Check sheet for the modelled part. Datum: model origin and axes. Units: mm. A direction names the side the tool comes from. Round coordinates to 2 decimals unless told otherwise and drop trailing zeros. Write each loop counter-clockwise with the first axis right and the second up, starting at its lowest first coordinate (ties: lowest second). Pieces come first, ordered by that corner, then holes.
Item 1: Cross-section at C-C on y = -2.5. Enter the section's corners in (x, z).
Item 2: Tool access check on faces 4 (the cylindrical face through (-0.867, -3.905, -0.246)), 5 (the flat face through (1.3, -1.3, 1)), 6 (the flat face through (2, 0, -0.5)). Record the directions out of +Z, -Z, +X, -X, +Y, -Y that give a thin tool (end or side, any length) a straight path to the whole face; none if there is none.
Item 3: Go/stop test with flat-tipped pins: pin 1 Ø1.5 at (x, z) = (3.5, 8.5) entering from -Y; pin 2 Ø3 at (x, y) = (1, -0.5) entering from +Z; pin 3 Ø2 at (x, z) = (4, 2.5) entering from -Y. Record where each tip stops, or that it passes through.
Item 4: Cross-section at A-A on y = -0.5. Enter the section's corners in (x, z), plus the area to 3 significant figures.
Item 5: Release check for a two-part mould opening along Y. For faces 1 (the cylindrical face through (-1.653, 2.593, 5.338)), 2 (the cylindrical face through (0, 5, 5)), 3 (the flat face through (0.1, 3.3, 9.8)) record: +Y half, -Y half, draft (parallel to the pull), parting line (faces both ways), or undercut.
Item 6: Material ranges on line 1 (Y direction, x = 0, z = 0.15); line 2 (Y direction, x = 0, z = -0.05), recorded low to high.
Autodesk Fusion 360 part; units mm, degrees
sketch "Sketch1" plane through (0, 0, 0) normal (0, 0, 1) x (1, 0, 0)
  circle A0 centre (0, 0) radius 5
  circle A1 centre (0, 0) radius 1.65
  dimension "d1" = 10
  dimension "d2" = 3.3
extrude "Extrude1" add sketch "Sketch1" along normal blind 1
sketch "Sketch2" plane through (0, 0, 1) normal (0, 0, 1) x (-1, 0, 0)
  circle A0 centre (0, 0) radius 1.65
  circle A1 centre (0, 0) radius 5
  circle A2 centre (0, 0) radius 3.075
  dimension "d5" = 6.15
extrude "Extrude2" add sketch "Sketch2" along normal blind 8.8 contours A1
sketch "Sketch3" plane through (0, 0, 0) normal (0, 0, -1) x (1, 0, 0)
  circle A0 centre (0, 0) radius 1.65
  circle A1 centre (0, 0) radius 5
  circle A2 centre (0, 0) radius 4
  dimension "d8" = 8
extrude "Extrude3" add sketch "Sketch3" along normal blind 0.5 contours A2
sketch "Sketch4" plane through (0, 0, 0) normal (0, 1, 0) x (1, 0, 0)
  ellipse E0 centre (0, -9.8) end of major axis (-1, -9.8) minor radius 5
  line L0 (1, -9.8) -> (-1, -9.8)
  line L1 (0, -4.8) -> (0, -14.8)
  line L2 (-5, -9.8) -> (5, -9.8)
  line L3 (-5, 0) -> (5, 0)
  dimension "d11" = 2
  dimension "d12" = 10
  dimension "d15" = 9.8
  dimension "d16" = 9.8
extrude "Extrude4" cut sketch "Sketch4" against normal blind 15
equation "d2 = 3 mm + 0.3 mm"
equation "d15 = d16"
Response values:
1. outline: (-4.33, 0) - (-3.12, 0) - (-3.12, -0.5) - (3.12, -0.5) - (3.12, 0) - (4.33, 0) - (4.33, 9.8) - (1.79, 9.8) - (1.79, 1) - (-1.79, 1) - (-1.79, 9.8) - (-4.33, 9.8) - close
2. face 4: -Z
2. face 5: +Z
2. face 6: -Z, +X, -X, +Y, -Y
3. pin 1: stops at y = -4.18
3. pin 2: stops at z = 1
3. pin 3: stops at y = -4
4. outline: (-4.97, 0) - (-3.97, 0) - (-3.97, -0.5) - (-1.57, -0.5) - (-1.57, 1) - (-3.03, 1) - (-3.03, 9.8) - (-4.97, 9.8) - close; (1.57, -0.5) - (3.97, -0.5) - (3.97, 0) - (4.97, 0) - (4.97, 9.8) - (3.03, 9.8) - (3.03, 1) - (1.57, 1) - close
4. area: 43.4 mm2
5. face 1: undercut
5. face 2: parting line
5. face 3: draft
6. line 1: y = -5 to -1.65, 1.65 to 5
6. line 2: y = -4 to -1.65, 1.65 to 4
